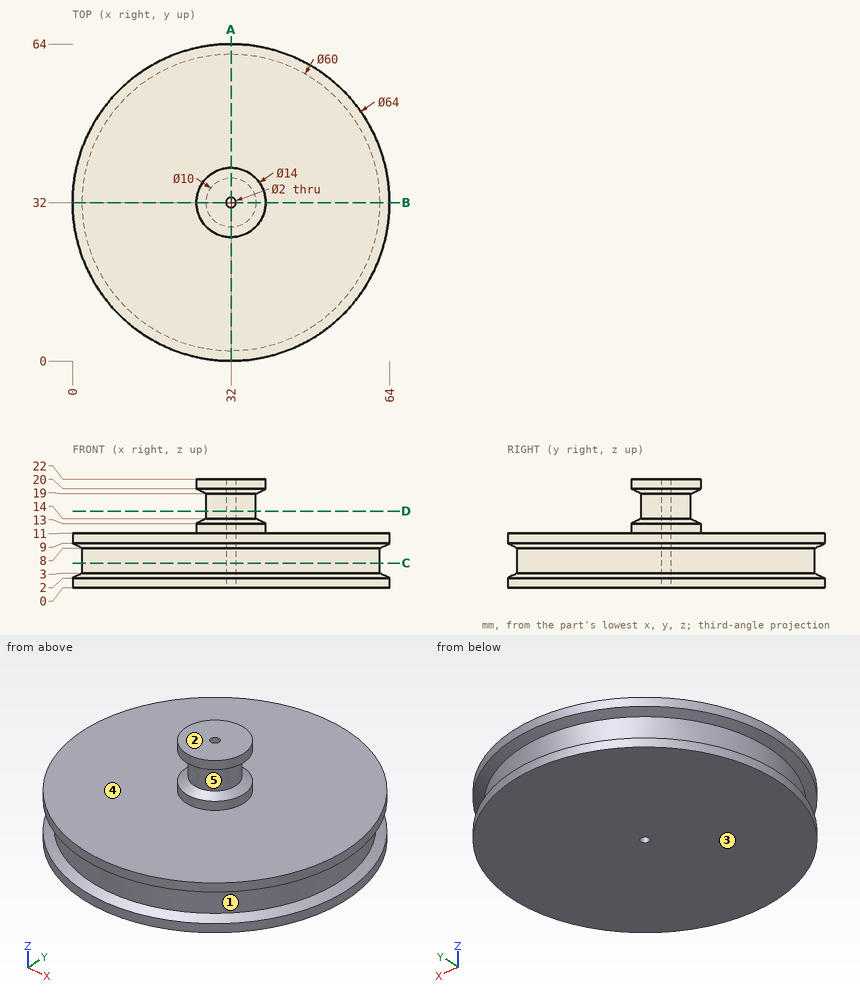
Check sheet for the drawn part. Datum: minimum x, y, z corner. Units: mm. A direction names the side the tool comes from. Round coordinates to 2 decimals unless told otherwise and drop trailing zeros. Write each loop counter-clockwise with the first axis right and the second up, starting at its lowest first coordinate (ties: lowest second). Pieces come first, ordered by that corner, then holes. Notation, with made-up numbers: (16.5, -28) -> (67.5, -28) arc R29 cw to (67.5, 6) -> close; hole circle Ø10 at (-18.75, 57.25). An arc over 180 degrees is marked (long way). Put each result on its own line as item: value.
(1) Go/stop test with flat-tipped pins: pin 1 Ø3 at (x, y) = (32.5, 56.5) entering from +Z; pin 2 Ø2 at (x, z) = (14, 9) entering from -Y; pin 3 Ø2 at (x, z) = (16, 5) entering from -Y. Record where each tip stops, or that it passes through.
Values found:
pin 1: stops at z = 11
pin 2: stops at y = 4.89
pin 3: stops at y = 6.02
(2) Sectioned sample at A-A (x = 32). Enter the section's corners in (y, z), plus the area to 3 significant figures.
Values found:
outline: (0, 0) -> (31, 0) -> (31, 22) -> (25, 22) -> (25, 20) -> (27, 19) -> (27, 14) -> (25, 13) -> (25, 11) -> (0, 11) -> (0, 9) -> (2, 8) -> (2, 3) -> (0, 2) -> close; (33, 0) -> (64, 0) -> (64, 2) -> (62, 3) -> (62, 8) -> (64, 9) -> (64, 11) -> (39, 11) -> (39, 13) -> (37, 14) -> (37, 19) -> (39, 20) -> (39, 22) -> (33, 22) -> close
area: 766 mm^2
(3) Tool access check on the marked faces 1 and 2. Record the directions out of +Z, -Z, +X, -X, +Y, -Y that give a thin tool (end or side, any length) a straight path to the whole face; none if there is none.
Values found:
face 1: none
face 2: +Z, +X, -X, +Y, -Y
(4) Sectioned sample at C-C (z = 5). Enter the section's corners in (x, y).
Values found:
outline: circle Ø60 at (32, 32); hole circle Ø2 at (32, 32)
(5) Material ranges on line 1 (Y direction, x = 32, z = 10.5); line 2 (Y direction, x = 32, z = 15); line 3 (Z direction, x = 22.5, y = 53.5), recorded low to high.
Values found:
line 1: y = 0 to 31, 33 to 64
line 2: y = 27 to 31, 33 to 37
line 3: z = 0 to 11
(6) Sectioned sample at D-D (z = 15.5). Enter the section's corners in (x, y).
Values found:
outline: circle Ø10 at (32, 32); hole circle Ø2 at (32, 32)
(7) Mould release check, pull along Z, two halves, no side actions. Record for the marked faces 3, 4 and 5: released by +Z, released by -Z, zero draft, split by the parting line, or undercut.
Values found:
face 3: released by -Z
face 4: released by +Z
face 5: undercut
